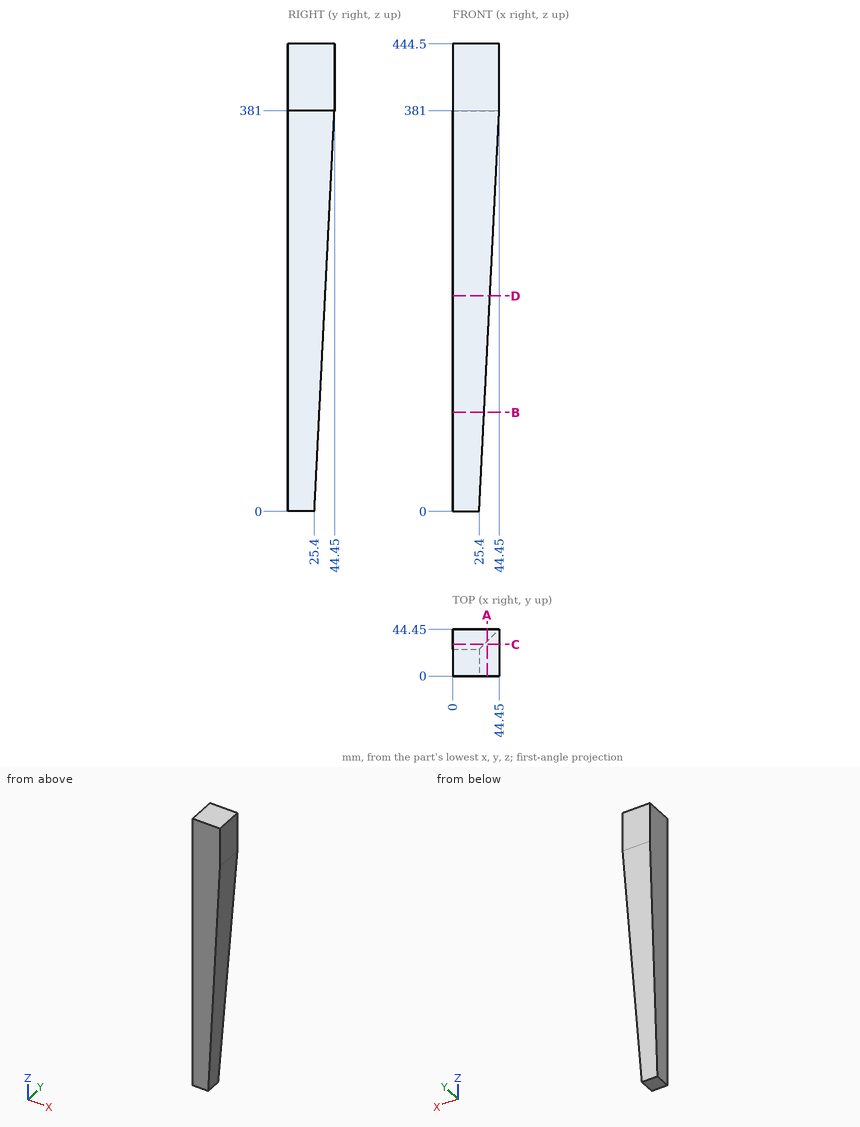
Input: dimensioned drawing with shaded views. Units: mm. Origin: part minimum x, y, z. Round coordinates to 2 decimals unless told otherwise and drop trailing zeros. Order: outer loops, then holes, each group sorted by start corner. A loop starts at its lowest first (then second) coordinate and runs counter-clockwise, first axis right, second up. Notation, with made-up numbers: (79.5, 66) -> (133.5, 66) arc R17 cw to (133.5, 71) -> close; hole circle Ø5 at (-35.5, 47). An arc over 180 degrees is marked (long way). One line per item, written item: value. Start each with the question number.
Q1. Section query A-A (x = 33). Return the cut outline in (y, z).
Q2. Section query B-B (z = 94). Return the cut outline in (x, y).
Q3. Material intervals for probe 1 along X at (y, z) = (33, 229); probe 2 along Y at (x, z) = (27, 45); probe 3 along X at (y, z) = (25, 226.5) (3 decimals), sorted ascending.
Q4. Pin query (flat end, axial travel): pin 1 (5 mm diameter, centred on x = 7, z = 294.5, fed in from -Y); pin 2 (1.5 mm diameter, centred on x = 12.5, z = 123, fed in from +Y); pin 3 (4 mm diameter, centred on y = 11, z = 188.5, fed in from +X) (3 decimals); pin 4 (1 mm diameter, centred on y = 17, z = 379.5, fed in from +X). Return the tip coordinate at first contact, or that it passes through.
Q5. Section query C-C (y = 30). Return the cut outline in (x, z), plus the area to 3 significant figures.
Q6. Section query D-D (z = 205). Return the cut outline in (x, y), plus the area to 3 significant figures.
Findings below:
1. outline: (0, 152) -> (33, 152) -> (44.45, 381) -> (44.45, 444.5) -> (0, 444.5) -> close
2. outline: (0, 0) -> (30.1, 0) -> (30.1, 30.1) -> (0, 30.1) -> close
3. probe 1: 0 to 36.85
3. probe 2: 0 to 27.65
3. probe 3: 0 to 36.725
4. pin 1: y = 0
4. pin 2: y = 31.59
4. pin 3: x = 34.925
4. pin 4: x = 44.4
5. outline: (0, 92) -> (30, 92) -> (44.45, 381) -> (44.45, 444.5) -> (0, 444.5) -> close
5. area: 13,600 mm²
6. outline: (0, 0) -> (35.65, 0) -> (35.65, 35.65) -> (0, 35.65) -> close
6. area: 1,270 mm²
